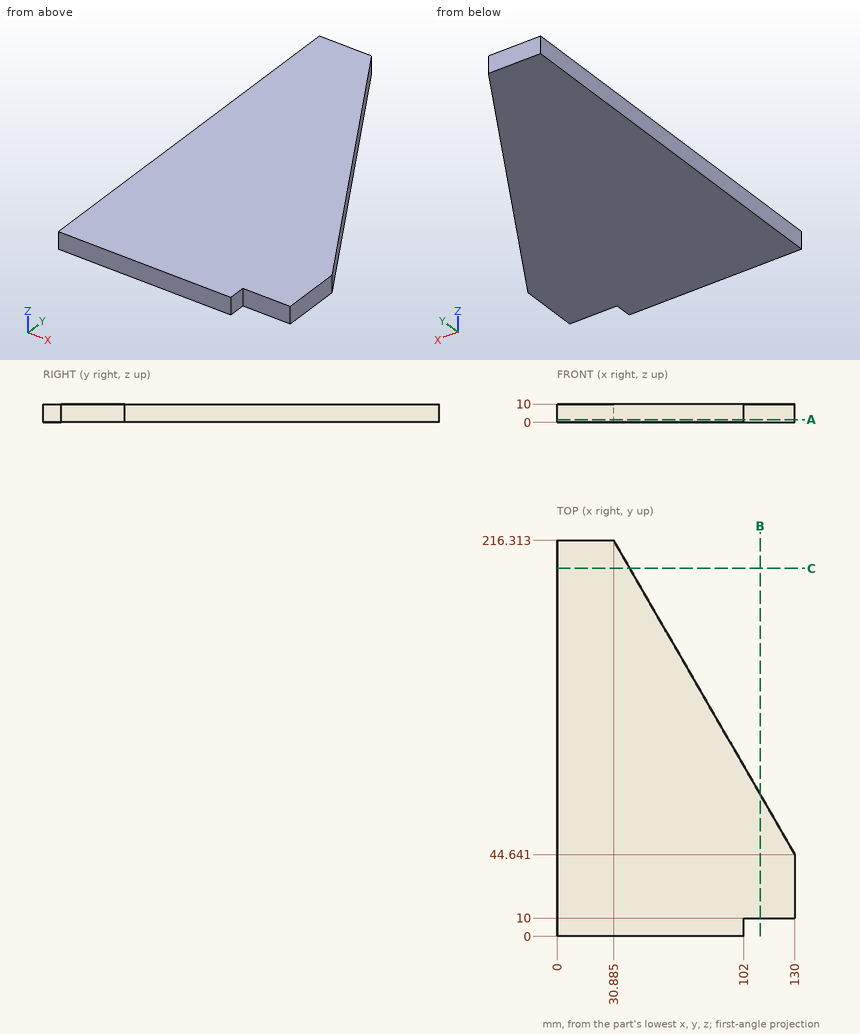
Job drawing, mm, ordinate dimensions from the low corner. One solid piece. Coordinates: 2 decimals unless noted, no trailing zeros. Order: outer loops, then holes, each group sorted by start corner. A loop starts at its lowest first (then second) coordinate and runs counter-clockwise, first axis right, second up. Notation, with made-up numbers: (76, -33.75) -> (132, -33.75) arc R27 cw to (132, -2.75) -> close; hole circle Ø7 at (74.25, 40.5). An arc over 180 degrees is marked (long way). Put each result on its own line as item: value. Start each with the question number.
(1) Band-saw the part on C-C (y = 201). Give the cut face in (x, z), then the cut area to 3 significant figures.
(2) Probe line 1 along Y through (x, z) = (116.5, 2) (1 decimal); line 2 along X through (y, z) = (200, 4.25) (1 decimal); line 3 along Y through (x, z) = (79, 8.25) (1 decimal). List the from-to ranges inside material, lowest first. Write a range as [from, to].
(3) Band-saw the part on B-B (x = 111). Give the cut face in (y, z).
(4) Pin check, flat tips, straight feed: pin 1 Ø4 at (y, z) = (156.5, 6.5) entering from -X; pin 2 Ø1.5 at (y, z) = (124.5, 7) entering from +X; pin 3 Ø6 at (x, z) = (93, 4.5) entering from +Y (1 decimal); pin 4 Ø5 at (y, z) = (6, 5.5) entering from +X. Stop position of each tip, or through.
(5) Band-saw the part on A-A (z = 1.5). Give the cut face in (x, y) (1 decimal), then the cut area to 3 significant figures.
Determined:
1. outline: (0, 0) -> (39.73, 0) -> (39.73, 10) -> (0, 10) -> close
1. area: 397 mm²
2. line 1: y = [10, 68]
2. line 2: x = [0, 40.3]
2. line 3: y = [0, 133]
3. outline: (10, 0) -> (77.55, 0) -> (77.55, 10) -> (10, 10) -> close
4. pin 1: stops at x = 0
4. pin 2: stops at x = 84.33
4. pin 3: stops at y = 113.9
4. pin 4: stops at x = 102
5. outline: (0, 0) -> (102, 0) -> (102, 10) -> (130, 10) -> (130, 44.6) -> (30.9, 216.3) -> (0, 216.3) -> close
5. area: 19,300 mm²
